Geometry check sheet. Reference: the model listing, model coordinates, mm. A direction names the side the tool comes from. Give positions to 0.01 mm unless a question says otherwise; leave off trailing zeros. Loops run counter-clockwise (first coordinate to the right, second up) from the corner with the lowest first, then second, coordinate; pieces in that order, holes last. Notation, with made-up numbers: (30, 29) -> (47, 29) arc R23 cw to (47, 43) -> close; hole circle Ø9 at (33, 70). An arc over 180 degrees is marked (long way). Answer as a JSON object with one key per item and string values.
from build123d import *

# Parameters (mm, degrees)
SKETCH_1_W          = 400
SKETCH_1_H          = 60
SKETCH_1_R          = 1.6
SKETCH_1_W_2        = 21
SKETCH_1_H_2        = 21
SKETCH_1_W_3        = 240
SKETCH_1_H_3        = 75
SKETCH_1_R_2        = 20
EXTRUDE_1484_DEPTH  = 3
SKETCH_2_R          = 2.05
SKETCH_2_R_2        = 2.1
CUT_EXTRUDE_1_DEPTH = 250.229009796
FILLET_1_R          = 5
SKETCH1_R           = 2.1
CUT_EXTRUDE4_DEPTH  = 250.229009796
CUT_EXTRUDE_2_DEPTH = 10
FILLET_2_R          = 5


with BuildPart() as part:
    # 草图1 → Extrude 1484 (new body)
    # profile 1 of 2: a face of its own
    with BuildSketch(Plane(origin=(0, 0, 0), x_dir=(1, 0, 0), z_dir=(0, 1, 0))):
        with Locations((32.825924772, 16.128249268)):
            Rectangle(SKETCH_1_W, SKETCH_1_H)
        with Locations(Location((-14.674075228, 36.128249268, 0), (0, 0, 270))):
            Circle(SKETCH_1_R, mode=Mode.SUBTRACT)
        with Locations(Location((-14.674075228, 11.128249268, 0), (0, 0, 270))):
            Circle(SKETCH_1_R, mode=Mode.SUBTRACT)
        with Locations(Location((80.325924772, 11.128249268, 0), (0, 0, 270))):
            Circle(SKETCH_1_R, mode=Mode.SUBTRACT)
        with Locations(Location((80.325924772, 36.128249268, 0), (0, 0, 270))):
            Circle(SKETCH_1_R, mode=Mode.SUBTRACT)
        with Locations((32.825924772, 10.628249268)):
            Rectangle(SKETCH_1_W_2, SKETCH_1_H_2, mode=Mode.SUBTRACT)
    # profile 2 of 2: a face of its own
    with BuildSketch(Plane(origin=(0, 0, 0), x_dir=(1, 0, 0), z_dir=(0, 1, 0))):
        with Locations((32.825924772, -51.371750732)):
            Rectangle(SKETCH_1_W_3, SKETCH_1_H_3)
        with Locations(Location((7.825924772, -29.871750732, 0), (0, 0, 270))):
            Circle(SKETCH_1_R, mode=Mode.SUBTRACT)
        with Locations(Location((7.825924772, -79.871750732, 0), (0, 0, 270))):
            Circle(SKETCH_1_R, mode=Mode.SUBTRACT)
        with Locations(Location((57.825924772, -79.871750732, 0), (0, 0, 270))):
            Circle(SKETCH_1_R, mode=Mode.SUBTRACT)
        with Locations(Location((57.825924772, -29.871750732, 0), (0, 0, 270))):
            Circle(SKETCH_1_R, mode=Mode.SUBTRACT)
        with Locations(Location((32.825924772, -54.871750732, 0), (0, 0, 270))):
            Circle(SKETCH_1_R_2, mode=Mode.SUBTRACT)
    extrude(amount=EXTRUDE_1484_DEPTH)

    # 草图2 → 切除-拉伸1 (cut, through all)
    with BuildSketch(Plane(origin=(0, 3, 0), x_dir=(1, 0, 0), z_dir=(0, 1, 0))):
        with Locations(Location((-149.174075228, 29.628249268, 0), (0, 0, 270))):
            Circle(SKETCH_2_R)
        with Locations(Location((-149.174075228, 2.628249268, 0), (0, 0, 270))):
            Circle(SKETCH_2_R)
        with Locations(Location((-121.674075228, 29.628249268, 0), (0, 0, 270))):
            Circle(SKETCH_2_R)
        with Locations(Location((-121.674075228, 2.628249268, 0), (0, 0, 90))):
            Circle(SKETCH_2_R)
        with Locations(Location((-51.674075228, 41.128249268, 0), (0, 0, 270))):
            Circle(SKETCH_2_R_2)
        with Locations(Location((-86.674075228, 41.128249268, 0), (0, 0, 270))):
            Circle(SKETCH_2_R_2)
        with Locations(Location((-51.674075228, -8.871750732, 0), (0, 0, 90))):
            Circle(SKETCH_2_R_2)
        with Locations(Location((-86.674075228, -8.871750732, 0), (0, 0, 90))):
            Circle(SKETCH_2_R_2)
        with Locations(Location((-135.424075228, 41.128249268, 0), (0, 0, 270))):
            Circle(SKETCH_2_R_2)
        with Locations(Location((-135.424075228, -8.871750732, 0), (0, 0, 90))):
            Circle(SKETCH_2_R_2)
        with Locations(Location((201.075924772, -8.871750732, 0), (0, 0, 270))):
            Circle(SKETCH_2_R_2)
        with Locations(Location((201.075924772, 41.128249268, 0), (0, 0, 90))):
            Circle(SKETCH_2_R_2)
        with Locations(Location((152.325924772, -8.871750732, 0), (0, 0, 270))):
            Circle(SKETCH_2_R_2)
        with Locations(Location((117.325924772, -8.871750732, 0), (0, 0, 270))):
            Circle(SKETCH_2_R_2)
        with Locations(Location((152.325924772, 41.128249268, 0), (0, 0, 90))):
            Circle(SKETCH_2_R_2)
        with Locations(Location((117.325924772, 41.128249268, 0), (0, 0, 90))):
            Circle(SKETCH_2_R_2)
        with Locations(Location((187.325924772, 2.628249268, 0), (0, 0, 270))):
            Circle(SKETCH_2_R)
        with Locations(Location((187.325924772, 29.628249268, 0), (0, 0, 90))):
            Circle(SKETCH_2_R)
        with Locations(Location((214.825924772, 2.628249268, 0), (0, 0, 90))):
            Circle(SKETCH_2_R)
        with Locations(Location((214.825924772, 29.628249268, 0), (0, 0, 90))):
            Circle(SKETCH_2_R)
    extrude(amount=-CUT_EXTRUDE_1_DEPTH, mode=Mode.SUBTRACT)

    # 圆角1
    fillet_1_edges = [part.edges().sort_by_distance(p)[0] for p in [
        (-167.174075228, 1.5, 13.871750732),
        (-167.174075228, 1.5, -46.128249268),
        (232.825924772, 1.5, -46.128249268),
        (232.825924772, 1.5, 13.871750732),
        (152.825924772, 1.5, 13.871750732),
        (152.825924772, 1.5, 88.871750732),
        (-87.174075228, 1.5, 88.871750732),
        (-87.174075228, 1.5, 13.871750732),
    ]]
    fillet(fillet_1_edges, radius=FILLET_1_R)

    # Sketch1 → Cut-Extrude4 (cut, through all)
    with BuildSketch(Plane(origin=(0, 0, 0), x_dir=(1, 0, 0), z_dir=(0, 1, 0))):
        with Locations(Location((-72.174075228, -33.871750732, 0), (0, 0, 270))):
            Circle(SKETCH1_R)
        with Locations(Location((-72.174075228, -68.871750732, 0), (0, 0, 270))):
            Circle(SKETCH1_R)
        with Locations(Location((137.825924772, -68.871750732, 0), (0, 0, 90))):
            Circle(SKETCH1_R)
        with Locations(Location((137.825924772, -33.871750732, 0), (0, 0, 90))):
            Circle(SKETCH1_R)
        with BuildLine():
            Line((-42.174075228, -68.871750732), (-42.174075228, -33.871750732))
            ThreePointArc((-42.174075228, -33.871750732), (-32.174075228, -23.871750732), (-22.174075228, -33.871750732))
            Line((-22.174075228, -33.871750732), (-22.174075228, -68.871750732))
            ThreePointArc((-22.174075228, -68.871750732), (-32.174075228, -78.871750732), (-42.174075228, -68.871750732))
        make_face()
        with BuildLine():
            Line((107.825924772, -68.871750732), (107.825924772, -33.871750732))
            ThreePointArc((107.825924772, -33.871750732), (97.825924772, -23.871750732), (87.825924772, -33.871750732))
            Line((87.825924772, -33.871750732), (87.825924772, -68.871750732))
            ThreePointArc((87.825924772, -68.871750732), (97.825924772, -78.871750732), (107.825924772, -68.871750732))
        make_face()
    extrude(amount=CUT_EXTRUDE4_DEPTH, mode=Mode.SUBTRACT)

    # 草图3 → 切除-拉伸2 (cut)
    with BuildSketch(Plane(origin=(0, 3, 0), x_dir=(1, 0, 0), z_dir=(0, 1, 0))):
        with BuildLine():
            Line((227.825924772, 46.128249268), (-162.174075228, 46.128249268))
            ThreePointArc((-162.174075228, 46.128249268), (-165.709609134, 44.663783174), (-167.174075228, 41.128249268))
            Line((-167.174075228, 41.128249268), (-167.174075228, -8.871750732))
            ThreePointArc((-167.174075228, -8.871750732), (-165.709609134, -12.407284637), (-162.174075228, -13.871750732))
            Line((-162.174075228, -13.871750732), (-92.174075228, -13.871750732))
            Line((-92.174075228, -13.871750732), (157.825924772, -13.871750732))
            Line((157.825924772, -13.871750732), (227.825924772, -13.871750732))
            ThreePointArc((227.825924772, -13.871750732), (231.361458678, -12.407284637), (232.825924772, -8.871750732))
            Line((232.825924772, -8.871750732), (232.825924772, 41.128249268))
            ThreePointArc((232.825924772, 41.128249268), (231.361458678, 44.663783174), (227.825924772, 46.128249268))
        make_face()
        with BuildLine():
            Line((-87.174075228, -13.871750732), (-92.174075228, -13.871750732))
            ThreePointArc((-92.174075228, -13.871750732), (-88.638541322, -15.336216826), (-87.174075228, -18.871750732))
            Line((-87.174075228, -18.871750732), (-87.174075228, -13.871750732))
        make_face()
        with BuildLine():
            Line((157.825924772, -13.871750732), (152.825924772, -13.871750732))
            Line((152.825924772, -13.871750732), (152.825924772, -18.871750732))
            ThreePointArc((152.825924772, -18.871750732), (154.290390866, -15.336216826), (157.825924772, -13.871750732))
        make_face()
    extrude(amount=-CUT_EXTRUDE_2_DEPTH, mode=Mode.SUBTRACT)

    # 圆角2
    fillet_2_edges = [part.edges().sort_by_distance(p)[0] for p in [
        (152.825924772, 1.5, 13.871750732),
        (-87.174075228, 1.5, 13.871750732),
    ]]
    fillet(fillet_2_edges, radius=FILLET_2_R)


solid = part.part
1) Section check C-C on z = 64. Record the cut outline in (x, y).
Geometry check:
{"outline": "(-87.17, 0) -> (-42.17, 0) -> (-42.17, 3) -> (-87.17, 3) -> close; (-22.17, 0) -> (15.03, 0) -> (15.03, 3) -> (-22.17, 3) -> close; (50.62, 0) -> (87.83, 0) -> (87.83, 3) -> (50.62, 3) -> close; (107.83, 0) -> (152.83, 0) -> (152.83, 3) -> (107.83, 3) -> close"}
2) Tool access check on faces 1 (the face through (97.61, 1.48, 78.87)), 2 (the face through (-85.748, 1.479, 15.375)). Record the directions out of +Z, -Z, +X, -X, +Y, -Y that give a thin tool (end or side, any length) a straight path to the whole face; none if there is none.
Geometry check:
{"face 1": "+Y, -Y", "face 2": "-Z, -X, +Y, -Y"}
3) Draft check along X on faces 3 (the face through (98.046, 1.479, 23.874)), 4 (the face through (151.4, 1.479, 15.375)), 5 (the face through (-85.748, 1.521, 87.368)). Enter one of: pulls with the +X half, pulls with the -X half, needs draft (parallel to the pull), parting line crosses it, or undercut.
Geometry check:
{"face 3": "undercut", "face 4": "pulls with the +X half", "face 5": "pulls with the -X half"}
4) Section check B-B on y = 2.5. Count the separate pieces of the cut face and the enclosed holes in it, plus the area to 3 significant figures.
Geometry check:
{"separate pieces": "1", "enclosed holes": "11", "area": "14,600 mm2"}
5) Section check A-A on z = 55. Record the cut outline in (x, y).
Geometry check:
{"outline": "(-87.17, 0) -> (-42.17, 0) -> (-42.17, 3) -> (-87.17, 3) -> close; (-22.17, 0) -> (12.83, 0) -> (12.83, 3) -> (-22.17, 3) -> close; (52.83, 0) -> (87.83, 0) -> (87.83, 3) -> (52.83, 3) -> close; (107.83, 0) -> (152.83, 0) -> (152.83, 3) -> (107.83, 3) -> close"}
6) Material ranges on line 1 along X through (y, z) = (0.6, 55); line 2 along X through (y, z) = (1.1, 56); line 3 along X through (y, z) = (1.25, 76), recorded low to high. Write a range as from..to.
Geometry check:
{"line 1": "x = -87.17..-42.17, -22.17..12.83, 52.83..87.83, 107.83..152.83", "line 2": "x = -87.17..-42.17, -22.17..12.86, 52.79..87.83, 107.83..152.83", "line 3": "x = -87.17..-39.19, -25.16..90.81, 104.84..152.83"}
